Build history of the part. All positions in model axes, mm. A direction names the side the tool comes from. Round coordinates to 2 decimals unless told otherwise and drop trailing zeros. Order: outer loops, then holes, each group sorted by start corner. A loop starts at its lowest first (then second) coordinate and runs counter-clockwise, first axis right, second up. Notation, with made-up numbers: (-40, 17) -> (-4, 17) arc R18 cw to (-4, 45) -> close; hole circle Ø8 at (75.5, 61). An arc over 180 degrees is marked (long way). Answer as CSV lines item,"result". Start each with the question number.
```python
from build123d import *

# Parameters (mm, degrees)
BOSS_EXTRUDE1_DEPTH = 6
FILLET1_R           = 10
SKETCH2_R           = 2.5
CUT_EXTRUDE1_DEPTH  = 6
SKETCH5_R           = 5.997593501
BOSS_EXTRUDE2_DEPTH = 6
FILLET2_R           = 10
SKETCH6_R           = 1.5
CUT_EXTRUDE2_DEPTH  = 10
SKETCH7_R           = 1.5
CUT_EXTRUDE3_DEPTH  = 10
SKETCH8_R           = 2
CUT_EXTRUDE4_DEPTH  = 10


with BuildPart() as part:
    # Sketch1 → Boss-Extrude1 (new body)
    with BuildSketch(Plane(origin=(0, 0, 0), x_dir=(1, 0, 0), z_dir=(0, 1, 0))):
        Polygon((21.213083016, -102.227633762), (35.213083016, -90.480238926), (35.213083016, -30.480238926), (21.213083016, -18.73284409), (21.213083016, 31.26715591), (35.213083016, 43.014550747), (35.213083016, 103.014550747), (-36.786916984, 103.014550747), (-36.786916984, 43.014550747), (-22.786916984, 31.26715591), (-22.786916984, -18.73284409), (-36.786916984, -30.480238926), (-36.786916984, -90.480238926), (-22.786916984, -102.227633762), align=None)
    extrude(amount=BOSS_EXTRUDE1_DEPTH)

    # Fillet1
    fillet1_edges = [part.edges().sort_by_distance(p)[0] for p in [
        (-22.786916984, 3, 102.227633762),
        (-36.786916984, 3, 90.480238926),
        (-36.786916984, 3, 30.480238926),
        (-22.786916984, 3, 18.73284409),
        (21.213083016, 3, 18.73284409),
        (35.213083016, 3, 30.480238926),
        (35.213083016, 3, 90.480238926),
        (21.213083016, 3, 102.227633762),
    ]]
    fillet(fillet1_edges, radius=FILLET1_R)

    # Sketch2 → Cut-Extrude1 (cut)
    with BuildSketch(Plane.XZ):
        with Locations(Location((-0.786916984, 60.480238926, 0), (0, 0, 270))):
            Circle(SKETCH2_R)
    extrude(amount=-CUT_EXTRUDE1_DEPTH, mode=Mode.SUBTRACT)

    # Sketch5 → Boss-Extrude2 (add)
    with BuildSketch(Plane.XZ):
        with Locations((-0.786916984, 60.480238926)):
            Circle(SKETCH5_R)
    extrude(amount=-BOSS_EXTRUDE2_DEPTH)

    # Fillet2
    fillet2_edges = [part.edges().sort_by_distance(p)[0] for p in [
        (-22.786916984, 3, -31.26715591),
        (-36.786916984, 3, -43.014550747),
        (35.213083016, 3, -43.014550747),
        (21.213083016, 3, -31.26715591),
    ]]
    fillet(fillet2_edges, radius=FILLET2_R)

    # Sketch6 → Cut-Extrude2 (cut)
    with BuildSketch(Plane(origin=(0, 6, 0), x_dir=(1, 0, 0), z_dir=(0, 1, 0))):
        with Locations(Location((15.213083016, 6.26715591, 0), (0, 0, 270))):
            Circle(SKETCH6_R)
        with Locations(Location((-16.786916984, 6.26715591, 0), (0, 0, 270))):
            Circle(SKETCH6_R)
    extrude(amount=-CUT_EXTRUDE2_DEPTH, mode=Mode.SUBTRACT)

    # Sketch7 → Cut-Extrude3 (cut)
    with BuildSketch(Plane(origin=(0, 6, 0), x_dir=(1, 0, 0), z_dir=(0, 1, 0))):
        with Locations(Location((20.993582106, -90.043344962, 0), (0, 0, 270))):
            Circle(SKETCH7_R)
        with Locations(Location((-22.567416075, -90.043344962, 0), (0, 0, 270))):
            Circle(SKETCH7_R)
    extrude(amount=-CUT_EXTRUDE3_DEPTH, mode=Mode.SUBTRACT)

    # Sketch8 → Cut-Extrude4 (cut)
    with BuildSketch(Plane(origin=(0, 0, 0), x_dir=(-1, 0, 0), z_dir=(0, -1, 0))):
        with Locations(Location((26.786916984, 73.014550747, 0), (0, 0, 90))):
            Circle(SKETCH8_R)
        with Locations(Location((-25.213083016, 73.014550747, 0), (0, 0, 90))):
            Circle(SKETCH8_R)
    extrude(amount=-CUT_EXTRUDE4_DEPTH, mode=Mode.SUBTRACT)


solid = part.part
```
Q1. Two-plate mould, pull along Z, no slides. Class faces 4 (the face through (26.565, 2.958, -71.54)), 5 (the face through (-1, 6, -2)), 6 (the face through (27.8, 3, 96.7)): +Z half, -Z half, draft (parallel to the pull), parting line (faces both ways), or undercut.
Q2. Slice it at A-A, the plane y = 2.9. Count the separate pieces of the cut face and the enclosed holes in it, plus the area to 3 significant figures.
Q3. Which spindle directions (+Z, -Z, +X, -X, +Y, -Y) get a long thin tool onto all of the face, cutting with end or side? Do faces 1 (the face through (-29.739, 2.958, 24.566)), 2 (the face through (22.12, 3.04, -30.77)), 3 (the face through (-25.435, 2.958, -71.54)). Say none if no direction does.
Q4. Probe L1, parallel to Z at x = 15, y = 1.7; L2, parallel to Z at x = 25, y = 2.35; L3, parallel to X at y = 2.4, z = -2. List the from-to ranges inside material, lowest first.
Q5. Slice it at B-B, the plane z = -18.5. Write the cut outline in (x, y).
Solutions:
1,face 4,"undercut"
1,face 5,"draft"
1,face 6,"+Z half"
2,separate pieces,"1"
2,enclosed holes,"6"
2,area,"12,800 mm2"
3,face 1,"-X, +Y, -Y"
3,face 2,"+X, +Y, -Y"
3,face 3,"+Y, -Y"
4,L1,"z = -103.01 to -7.75, -4.78 to 102.23"
4,L2,"z = -103.01 to -75, -71.03 to -34.44, 21.91 to 99.05"
4,L3,"x = -22.79 to 21.21"
5,outline,"(-22.79, 0) -> (21.21, 0) -> (21.21, 6) -> (-22.79, 6) -> close"
